Read the model definition and answer for the solid it produces. Units are mm, in the model's axes. A direction names the side the tool comes from. Round coordinates to 2 decimals unless told otherwise and drop trailing zeros. Write each loop counter-clockwise with the first axis right and the second up, starting at its lowest first coordinate (ties: lowest second). Pieces come first, ordered by that corner, then holes. Notation, with made-up numbers: (-1.5, 62.5) - (34.5, 62.5) arc R25 cw to (34.5, 93.5) - close; hole circle Ø3 at (88, 47). An arc over 180 degrees is marked (long way). Answer as CSV lines item,"result". Start each with the question number.
1) For a pull along Y with two mould halves and no side action, classify faces 1 (the cylindrical face through (-0.1, -4.84, 9.27)), 2 (the cylindrical face through (0.06, -2.87, 10.83)), 3 (the cylindrical face through (0.1, 4.84, 9.27)), 4 (the flat face through (5, 0, 6.4)) as +Y half, -Y half, draft (parallel to the pull), parting line (faces both ways), or undercut.
2) Consider line 1 along X through (y, z) = (0, 11); line 2 along X through (y, z) = (2, 3.5); line 3 along X through (y, z) = (-3, 10). Determine where each line is inside the solid, lowest interval first.
3) Which of the six approach directions +Z, -Z, +X, -X, +Y, -Y give full straight-line access (tool end or side, diameter ignored) to faces 5 (the flat face through (3, 0, 12.22)), 6 (the cylindrical face through (-0.06, 2.87, 10.83))?
4) Find section B-B on z = 6.75. Determine the outline of the cut face in (x, y).
5) Each of these flat-tipped pins is pushed along its axis until it touches: pin 1 (6 mm diameter, centred on y = -7.5, z = 9.5, fed in from -X); pin 2 (2 mm diameter, centred on y = 4.5, z = 6.5, fed in from -X); pin 3 (1.6 mm diameter, centred on x = -1, y = 0.5, fed in from +Z). Where does it stop, or does it pass through?
6) Find section A-A on z = 11.25. Determine the outline of the cut face in (x, y).
from build123d import *

# Parameters (mm, degrees)
F3_DEPTH = 5.82
F5_DEPTH = 7.75
F6_DEPTH = 5


with BuildPart() as f1:
    # F0 (on Front) → F1 (revolve)
    with BuildSketch(Plane.XZ):
        with BuildLine():
            Line((0, 6.4), (0, 0))
            ThreePointArc((0, 0), (6.668021, 1.704556), (11.7, 6.4))
            Line((11.7, 6.4), (0, 6.4))
        make_face()
    revolve(axis=Axis((0, 0, 3.2), (0, 0, 1)))

    # F2 (on face) → F3 (join)
    with BuildSketch(Plane.XY.offset(6.4)):
        with BuildLine():
            Line((4.65, -0.19), (4.65, 0.19))
            ThreePointArc((4.65, 0.19), (0, 4.84), (-4.65, 0.19))
            Line((-4.65, 0.19), (-4.65, -0.19))
            ThreePointArc((-4.65, -0.19), (0, -4.84), (4.65, -0.19))
        make_face()
        with BuildLine():
            Line((-2.68, -0.19), (-2.68, 0.19))
            ThreePointArc((-2.68, 0.19), (0, 2.87), (2.68, 0.19))
            Line((2.68, 0.19), (2.68, -0.19))
            ThreePointArc((2.68, -0.19), (0, -2.87), (-2.68, -0.19))
        make_face(mode=Mode.SUBTRACT)
    extrude(amount=F3_DEPTH)

    # F4 (on face) → F5 (cut)
    with BuildSketch(Plane.XY.offset(12.22)):
        with BuildLine():
            ThreePointArc((2.68, 0.19), (0, 2.87), (-2.68, 0.19))
            Line((-2.68, 0.19), (-2.68, -0.19))
            ThreePointArc((-2.68, -0.19), (0, -2.87), (2.68, -0.19))
            Line((2.68, -0.19), (2.68, 0.19))
        make_face()
    extrude(amount=-F5_DEPTH, mode=Mode.SUBTRACT)

    # F5_face (on face) → F6 (join)
    with BuildSketch(Plane.XY.offset(4.47)):
        with BuildLine():
            ThreePointArc((2.68, 0.19), (0, 2.87), (-2.68, 0.19))
            Line((-2.68, 0.19), (-2.68, -0.19))
            ThreePointArc((-2.68, -0.19), (0, -2.87), (2.68, -0.19))
            Line((2.68, -0.19), (2.68, 0.19))
        make_face()
    extrude(amount=F6_DEPTH)


solid = f1.part
Check values:
1,face 1,"-Y half"
1,face 2,"undercut"
1,face 3,"+Y half"
1,face 4,"draft"
2,line 1,"x = -4.65 to -2.68, 2.68 to 4.65"
2,line 2,"x = -9 to 9"
2,line 3,"x = -3.7 to 3.7"
3,face 5,"+Z, +X, -X, +Y, -Y"
3,face 6,"+Z"
4,outline,"(-4.65, -0.19) arc R4.65 ccw to (4.65, -0.19) - (4.65, 0.19) arc R4.65 ccw to (-4.65, 0.19) - close"
5,pin 1,"stops at x = -1.75"
5,pin 2,"stops at x = -11.16"
5,pin 3,"stops at z = 9.47"
6,outline,"(-4.65, -0.19) arc R4.65 ccw to (4.65, -0.19) - (4.65, 0.19) arc R4.65 ccw to (-4.65, 0.19) - close; hole (-2.68, -0.19) arc R2.68 ccw to (2.68, -0.19) - (2.68, 0.19) arc R2.68 ccw to (-2.68, 0.19) - close"
